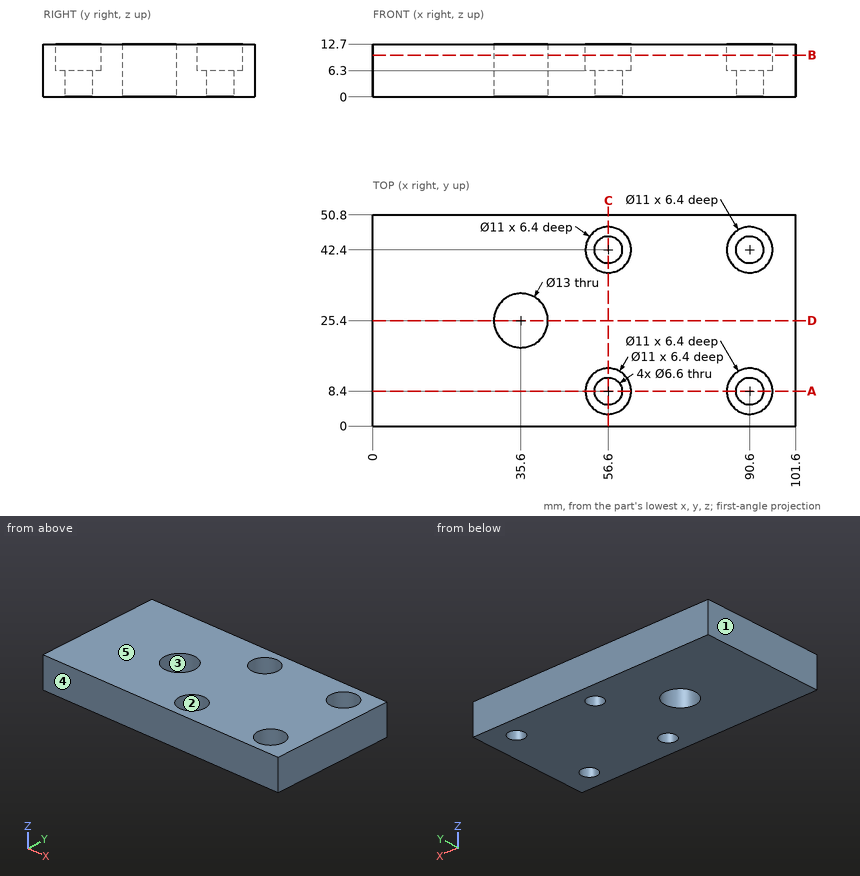
Geometry check sheet. Reference: drawing and pictorial views, mm from the part's lowest x, y, z. A direction names the side the tool comes from. Coordinates: 2 decimals unless noted, no trailing zeros. Order: outer loops, then holes, each group sorted by start corner. A loop starts at its lowest first (then second) coordinate and runs counter-clockwise, first axis right, second up. Notation, with made-up numbers: (54, -31.75) -> (70, -31.75) arc R12 ccw to (70, -16.75) -> close; hole circle Ø1 at (83, 39.5). An arc over 180 degrees is marked (long way). Use CSV: the item, a comma, the result in double quotes. Start each with the question number.
Q1. Tool access check on the marked faces 1 and 2. Record the directions out of +Z, -Z, +X, -X, +Y, -Y that give a thin tool (end or side, any length) a straight path to the whole face; none if there is none.
Q2. Section check B-B, the plane z = 10. Record the cut outline in (x, y), and give its area (3 significant figures).
Q3. Depth check by flat-ended pin: P1, Ø10.5, axis at x = 35.6, y = 25.4, coming from the +Z side; P2, Ø9, axis at x = 90.6, y = 42.4, coming from the +Z side. Enter the tip coordinate at first touch or a pass-through.
Q4. Section check D-D, the plane y = 25.4. Record the cut outline in (x, z).
Q5. Draft check along Y on the marked faces 3, 4 and 5. Enter one of: +Y half, -Y half, draft (parallel to the pull), parting line (faces both ways), or undercut.
Q6. Thickness scan on line 1 along Y through (x, z) = (56.6, 8.5); line 2 along Y through (x, z) = (56.6, 3.5); line 3 along X through (y, z) = (8.5, 2.25). Record the ranges inside material, lowest first.
Q7. Section check C-C, the plane x = 56.6. Record the cut outline in (y, z), and give its area (3 significant figures).
Q8. Section check A-A, the plane y = 8.4. Record the cut outline in (x, z), and give its area (3 significant figures).
Returned:
1,face 1,"+Z, -Z, -X, +Y, -Y"
1,face 2,"+Z"
2,outline,"(0, 0) -> (101.6, 0) -> (101.6, 50.8) -> (0, 50.8) -> close; hole circle Ø13 at (35.6, 25.4); hole circle Ø11 at (56.6, 8.4); hole circle Ø11 at (56.6, 42.4); hole circle Ø11 at (90.6, 8.4); hole circle Ø11 at (90.6, 42.4)"
2,area,"4,650 mm^2"
3,P1,"passes through"
3,P2,"stops at z = 6.3"
4,outline,"(0, 0) -> (29.1, 0) -> (29.1, 12.7) -> (0, 12.7) -> close; (42.1, 0) -> (101.6, 0) -> (101.6, 12.7) -> (42.1, 12.7) -> close"
5,face 3,"undercut"
5,face 4,"-Y half"
5,face 5,"draft"
6,line 1,"y = 0 to 2.9, 13.9 to 36.9, 47.9 to 50.8"
6,line 2,"y = 0 to 5.1, 11.7 to 39.1, 45.7 to 50.8"
6,line 3,"x = 0 to 53.3, 59.9 to 87.3, 93.9 to 101.6"
7,outline,"(0, 0) -> (5.1, 0) -> (5.1, 6.3) -> (2.9, 6.3) -> (2.9, 12.7) -> (0, 12.7) -> close; (11.7, 0) -> (39.1, 0) -> (39.1, 6.3) -> (36.9, 6.3) -> (36.9, 12.7) -> (13.9, 12.7) -> (13.9, 6.3) -> (11.7, 6.3) -> close; (45.7, 0) -> (50.8, 0) -> (50.8, 12.7) -> (47.9, 12.7) -> (47.9, 6.3) -> (45.7, 6.3) -> close"
7,area,"421 mm^2"
8,outline,"(0, 0) -> (53.3, 0) -> (53.3, 6.3) -> (51.1, 6.3) -> (51.1, 12.7) -> (0, 12.7) -> close; (59.9, 0) -> (87.3, 0) -> (87.3, 6.3) -> (85.1, 6.3) -> (85.1, 12.7) -> (62.1, 12.7) -> (62.1, 6.3) -> (59.9, 6.3) -> close; (93.9, 0) -> (101.6, 0) -> (101.6, 12.7) -> (96.1, 12.7) -> (96.1, 6.3) -> (93.9, 6.3) -> close"
8,area,"1,070 mm^2"
